Verification items for this drawing (mm, ordinates from the low corner). A direction names the side the tool comes from. Round coordinates to 2 decimals unless told otherwise and drop trailing zeros. Loops run counter-clockwise (first coordinate to the right, second up) from the corner with the lowest first, then second, coordinate; pieces in that order, holes last. Notation, with made-up numbers: (-2.75, 88) -> (56.25, 88) arc R29 ccw to (56.25, 111) -> close; hole circle Ø2 at (56, 77.25). An arc over 180 degrees is marked (long way). One line per item, written item: value. Start each with the question number.
1. Material ranges on L1, parallel to X at y = 3.25, z = 30; L2, parallel to X at y = 0.75, z = 25; L3, parallel to Z at x = 23, y = 2.5 (1 decimal), recorded low to high.
2. Cross-section at C-C on y = 2.5. Record the cut outline in (x, z).
3. Set-up check for the marked faces 1 and 2: record each of +Z, -Z, +X, -X, +Y, -Y from which the full face is reachable in a straight line by a thin tool's end or side.
4. Release check for a two-part mould opening along Z. For the marked faces 3, 4 and 5 record: +Z half, -Z half, draft (parallel to the pull), parting line (faces both ways), or undercut.
5. Cross-section at B-B on z = 7. Record the cut outline in (x, y) (1 decimal).
6. Cross-section at A-A on x = 34. Record the cut outline in (y, z) (1 decimal).
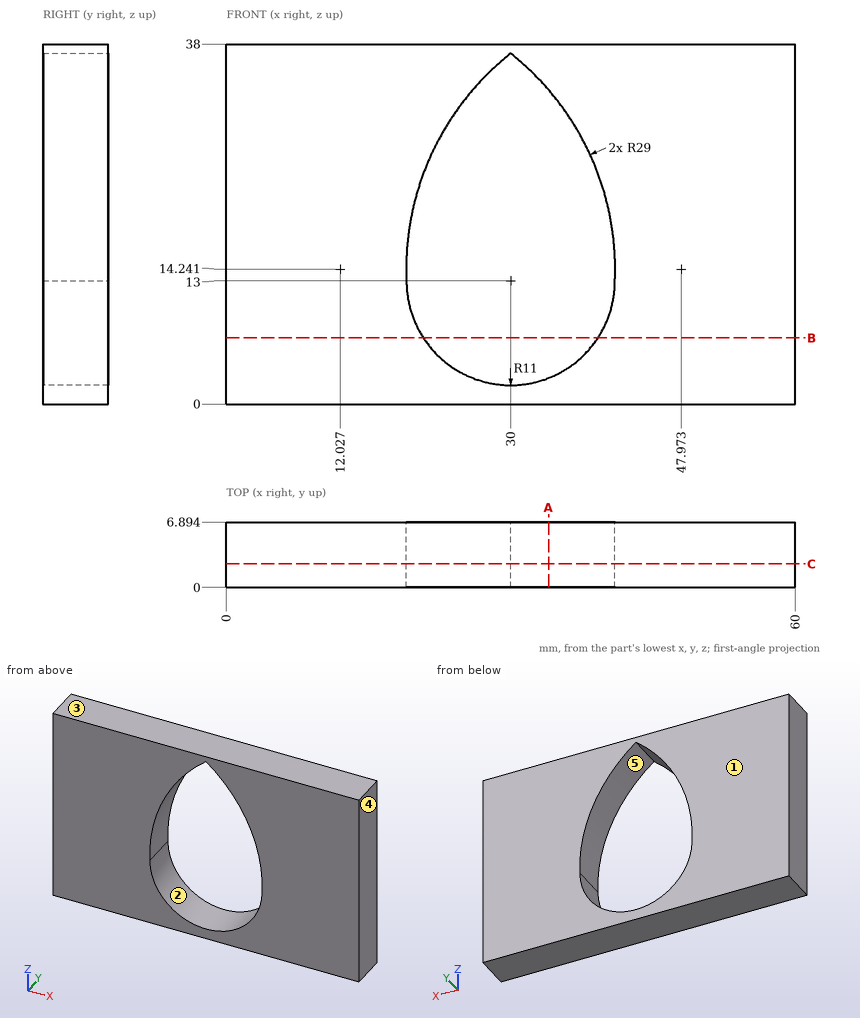
Taken from the geometry:
1. L1: x = 0 to 23.63, 36.37 to 60
1. L2: x = 0 to 21.04, 38.96 to 60
1. L3: z = 0 to 4.5, 29 to 38
2. outline: (0, 0) -> (60, 0) -> (60, 38) -> (0, 38) -> close; hole (19, 13) arc R11 ccw to (41, 13) arc R29 ccw to (30, 37) arc R29 ccw to start
3. face 1: +Z, -Z, +X, -X, +Y
3. face 2: +Y, -Y
4. face 3: +Z half
4. face 4: draft
4. face 5: undercut
5. outline: (0, 0) -> (20.8, 0) -> (20.8, 6.9) -> (0, 6.9) -> close; (39.2, 0) -> (60, 0) -> (60, 6.9) -> (39.2, 6.9) -> close
6. outline: (0, 0) -> (6.9, 0) -> (6.9, 2.8) -> (0, 2.8) -> close; (0, 33.2) -> (6.9, 33.2) -> (6.9, 38) -> (0, 38) -> close
